The model under review builds one solid part; all positions refer to its coordinate system, in mm. Face numbers are marked on the shaded views. A direction names the side the tool comes from. Coordinates: 2 decimals unless noted, no trailing zeros. Write each loop counter-clockwise with the first axis right and the second up, starting at its lowest first coordinate (ties: lowest second). Pieces come first, ordered by that corner, then holes. Notation, with made-up numbers: (87.5, 19) - (121.5, 19) arc R29 ccw to (121.5, 56) - close; hole circle Ø2 at (13, 38.5). An arc over 180 degrees is marked (long way). Put each result on its own line as item: value. Start each with the question number.
Item 1: Mouldability with a two-part tool opening along Y and no side actions: class the marked faces 3, 4 and 5 as pulls with the +Y half, pulls with the -Y half, needs draft (parallel to the pull), parting line crosses it, or undercut.
Item 2: Consider section C-C on z = 3.5. Give the boundary of the cut face in (x, y), then the cut area to 3 significant figures.
Item 3: For pin 1 (1 mm diameter, centred on x = -5, y = 3, fed in from +Z); pin 2 (1 mm diameter, centred on y = 4, z = 3.5, fed in from +X), all flat-tipped, find the tip position at first contact; note any pin that passes through.
Item 4: Consider section A-A on x = 0. Give the boundary of the cut face in (y, z), then the cut area to 3 significant figures.
Item 5: Machinability: for the marked faces 1 and 2, which of the approach directions +Z, -Z, +X, -X, +Y, -Y give a long, thin tool a straight path to every point of the face, cutting with its end or side? Answer none if there is none.
Item 6: To check wall thickness, follow L1, parallel to Y at x = 0, z = 0.45; L2, parallel to Y at x = 0, z = 5.05; L3, parallel to X at y = -2.5, z = 1.75. State the ranges of each line that lie inside material, in increasing order. Write a range as [from, to].
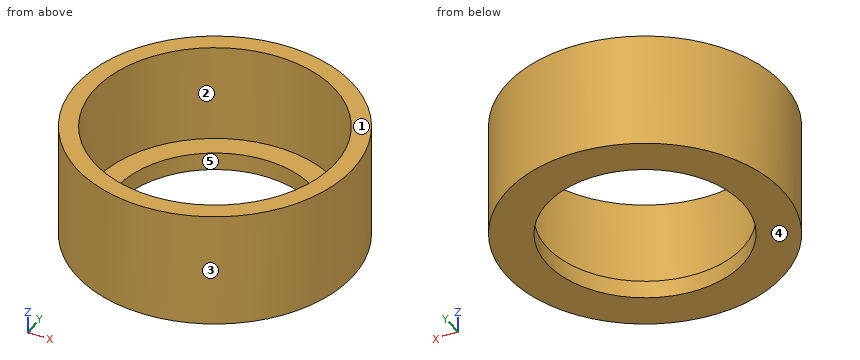
Autodesk Inventor part; units mm, degrees
ref_plane "YZ Plane" through (0, 0, 0) normal (1, 0, 0) x (0, 1, 0)
ref_plane "XZ Plane" through (0, 0, 0) normal (0, 1, 0) x (-1, 0, 0)
ref_plane "XY Plane" through (0, 0, 0) normal (0, 0, 1) x (1, 0, 0)
sketch "Sketch1" plane through (0, 0, 0) normal (0, 0, 1) x (1, 0, 0)
  circle A0 centre (0, 0) radius 6.75
  circle A1 centre (0, 0) radius 7.75
  dimension "d0" = 13.5
  dimension "d1" = 15.5
extrude "Extrusion1" add sketch "Sketch1" along normal blind 6.5
sketch "Sketch2" plane through (0, 0, 0) normal (0, 0, 1) x (1, 0, 0)
  circle A0 centre (0, 0) radius 6.75
  dimension "d4" = 13.5
extrude "Extrusion2" add sketch "Sketch2" along normal blind 1
sketch "Sketch3" plane through (0, 0, 1) normal (0, 0, 1) x (1, 0, 0)
  circle A0 centre (0, 0) radius 5.5
  dimension "d7" = 11
extrude "Extrusion3" cut sketch "Sketch3" against normal blind 1
properties part number "HubTest13mm"
Report:
1. face 3: parting line crosses it
1. face 4: needs draft
1. face 5: undercut
2. outline: circle Ø15.5 at (0, 0); hole circle Ø13.5 at (0, 0)
2. area: 45.6 mm²
3. pin 1: z = 1
3. pin 2: x = 6.91
4. outline: (-7.75, 0) - (-5.5, 0) - (-5.5, 1) - (-6.75, 1) - (-6.75, 6.5) - (-7.75, 6.5) - close; (5.5, 0) - (7.75, 0) - (7.75, 6.5) - (6.75, 6.5) - (6.75, 1) - (5.5, 1) - close
4. area: 15.5 mm²
5. face 1: +Z, +X, -X, +Y, -Y
5. face 2: +Z
6. L1: [-7.75, -5.5], [5.5, 7.75]
6. L2: [-7.75, -6.75], [6.75, 7.75]
6. L3: [-7.34, -6.27], [6.27, 7.34]
